Design review of the part shown in the three views and the two pictorial views. Dimensions are in mm from the part's minimum x, y and z. Coordinates: 2 decimals unless noted, no trailing zeros. Loops run counter-clockwise (first coordinate to the right, second up) from the corner with the lowest first, then second, coordinate; pieces in that order, holes last. Notation, with made-up numbers: (-31.5, 16) - (-5.5, 16) arc R26 ccw to (-5.5, 40) - close; hole circle Ø4 at (33.5, 85.5). An arc over 180 degrees is marked (long way). One line per item, written item: value. Start each with the question number.
1. To check wall thickness, follow line 1 (Y direction, x = 19.05, z = 15); line 2 (Y direction, x = 19.05, z = 5.75) (3 decimals); line 3 (X direction, y = 19.5, z = 15). State the ranges of each line that lie inside material, in increasing order. Write a range as from..to.
2. Take a section at C-C, the plane z = 9.5. State the section outline as (x, y) points (3 decimals), and give its area (3 significant figures).
3. Take a section at B-B, the plane y = 24. State the section outline as (x, z) points, and give its area (3 significant figures).
4. The part is to be moulded in two halves that separate along Z. For the marked faces 1, 2 and 3, say which applies: released by +Z, released by -Z, zero draft, split by the parting line, or undercut.
5. Take a section at A-A, the plane x = 19.05. State the section outline as (y, z) points (3 decimals).
6. Insertion check: pin 1 (8 mm diameter, centred on y = 14, z = 8.5, fed in from +X); pin 2 (2 mm diameter, centred on y = 18.5, z = 16, fed in from +X); pin 3 (2 mm diameter, centred on y = 8, z = 18.5, fed in from +X); pin 4 (6 mm diameter, centred on y = 32, z = 16.5, fed in from +X) (3 decimals). Each pin has a flat end and moves straight along its axis. Give the tip position at first contact, or say it passes through.
7. Take a section at D-D, the plane x = 11. State the section outline as (y, z) points, and give its area (3 significant figures).
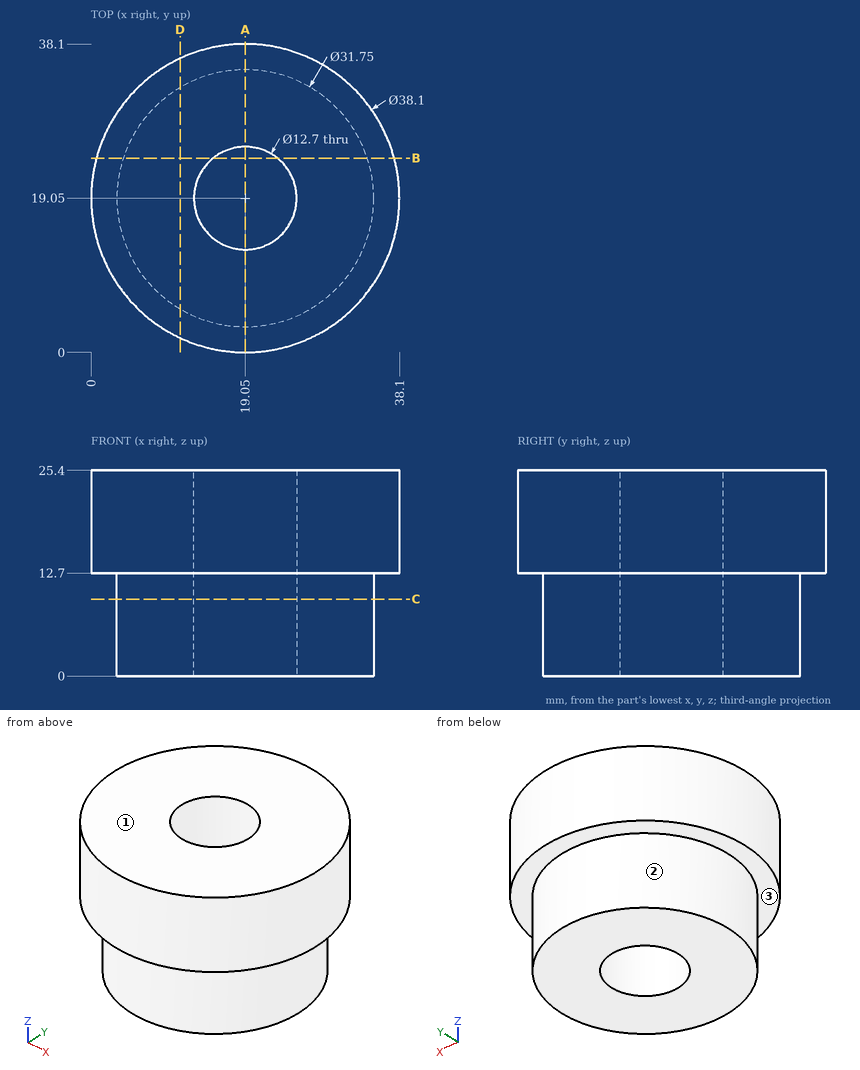
Solutions:
1. line 1: 0..12.7, 25.4..38.1
1. line 2: 3.175..12.7, 25.4..34.925
1. line 3: 0.01..12.72, 25.38..38.09
2. outline: circle Ø31.75 at (19.05, 19.05); hole circle Ø12.7 at (19.05, 19.05)
2. area: 665 mm2
3. outline: (0.65, 12.7) - (3.97, 12.7) - (3.97, 0) - (15.07, 0) - (15.07, 25.4) - (0.65, 25.4) - close; (23.03, 0) - (34.13, 0) - (34.13, 12.7) - (37.45, 12.7) - (37.45, 25.4) - (23.03, 25.4) - close
3. area: 648 mm2
4. face 1: released by +Z
4. face 2: zero draft
4. face 3: released by -Z
5. outline: (0, 12.7) - (3.175, 12.7) - (3.175, 0) - (12.7, 0) - (12.7, 25.4) - (0, 25.4) - close; (25.4, 0) - (34.925, 0) - (34.925, 12.7) - (38.1, 12.7) - (38.1, 25.4) - (25.4, 25.4) - close
6. pin 1: x = 34.89
6. pin 2: x = 38.1
6. pin 3: x = 35.23
6. pin 4: x = 35.295
7. outline: (1.78, 12.7) - (5.37, 12.7) - (5.37, 0) - (32.73, 0) - (32.73, 12.7) - (36.32, 12.7) - (36.32, 25.4) - (1.78, 25.4) - close
7. area: 786 mm2
